Design review of the part built by this model. Coordinates are the model's own, in mm. A direction names the side the tool comes from. Coordinates: 2 decimals unless noted, no trailing zeros. Loops run counter-clockwise (first coordinate to the right, second up) from the corner with the lowest first, then second, coordinate; pieces in that order, holes last. Notation, with made-up numbers: M -31,-9 L 16,-9 A30 ccw 16,14 Z; hole C 9.5,-25.75 d11. An arc over 180 degrees is marked long. Answer as a JSON object with one key per item and string values. Group by question number.
1. Consider section B-B (z = -2.5). State the section outline as (x, y) points, then the cut area to 3 significant figures.
2. Consider section A-A (x = -17.5). State the section outline as (y, z) points.
3. To check wall thickness, follow probe 1 along X at (y, z) = (-2, -1); probe 2 along Y at (x, z) = (-17.5, -2.3); probe 3 along Z at (x, y) = (13.5, -1.25). State the ranges of each line that lie inside material, in increasing order.
4. Draft analysis for pull direction X (two halves, no side actions). For faces 1 (the flat face through (23, 0, -2)), 2 (the flat face through (-11, 1, -2)), 3 (the flat face through (20, 0, 0)), state which applies: +X half, -X half, draft (parallel to the pull), parting line (faces both ways), or undercut.
5. Insertion check: pin 1 (4.5 mm diameter, centred on x = -17.5, y = 0, fed in from -Z); pin 2 (6 mm diameter, centred on x = -16, y = -1, fed in from +Z); pin 3 (1.5 mm diameter, centred on y = -4.5, z = 1.5, fed in from +X); pin 4 (1.5 mm diameter, centred on x = 4, y = 1.5, fed in from -Z). Each pin has a flat end and moves straight along its axis. Give the tip position at first contact, or say it passes through.
6. Consider section C-C (y = 0). Count the separate pieces of the cut face and the enclosed holes in it, then the cut area to 3 significant figures.
7. Machinability: for faces 4 (the flat face through (5.432, 0.158, 1.755)), 5 (the flat face through (0, 0, 4)), 6 (the flat face through (-11, 4, -3)), 7 (the flat face through (0, -6.8, 3)), 8 (the flat face through (-8.25, -5, -1)), which of the approach directions +Z, -Z, +X, -X, +Y, -Y give a long, thin tool a straight path to every point of the face, cutting with its end or side? Answer none if there is none.
from build123d import *

# Parameters (mm, degrees)
SKETCH_W        = 46
SKETCH_H        = 13.6
SKETCH_R        = 1.7
PAD_DEPTH       = 4
PAD001_DEPTH    = 4
SKETCH002_W     = 4.3
SKETCH002_H     = 1.7
POCKET_DEPTH    = 10
SKETCH003_W     = 16.5
SKETCH003_H     = 7.2
POCKET001_DEPTH = 4
SKETCH004_W     = 3
SKETCH004_H     = 1.5
POCKET002_DEPTH = 110.862709
SKETCH005_W     = 18.5
SKETCH005_H     = 3.5
SKETCH005_W_2   = 2.5
SKETCH005_H_2   = 6
POCKET003_DEPTH = 2
CHAMFER_SIZE    = 1.99
CHAMFER001_SIZE = 1.99


with BuildPart() as part:
    # Sketch → Pad (new body)
    with BuildSketch(Plane.XY):
        Rectangle(SKETCH_W, SKETCH_H)
        with Locations((-17.5, 0)):
            Circle(SKETCH_R, mode=Mode.SUBTRACT)
        with Locations((17.5, 0)):
            Circle(SKETCH_R, mode=Mode.SUBTRACT)
    extrude(amount=-PAD_DEPTH)

    # Sketch001 → Pad001 (new body)
    with BuildSketch(Plane.XY):
        with BuildLine():
            ThreePointArc((-4.75, 6.8), (-11.55, 0), (-4.75, -6.8))
            Line((-4.75, -6.8), (4.75, -6.8))
            ThreePointArc((4.75, -6.8), (11.55, 0), (4.75, 6.8))
            Line((-4.75, 6.8), (4.75, 6.8))
        make_face()
    extrude(amount=PAD001_DEPTH)

    # Sketch002 → Pocket (cut)
    with BuildSketch(Plane.XZ.offset(6.8)):
        Polygon((-7.588114, 2.079739), (-3.336138, 1.438879), (-3.589501, -0.242134), (-7.841477, 0.398725), align=None)
        with Locations((0, 0.5)):
            Rectangle(SKETCH002_W, SKETCH002_H)
        Polygon((3.336139, 1.438884), (7.588117, 2.079734), (7.841476, 0.39872), (3.589499, -0.24213), align=None)
    extrude(amount=-POCKET_DEPTH, mode=Mode.SUBTRACT)

    # Sketch003 → Pocket001 (cut)
    with BuildSketch(Plane.XZ.offset(6.8)):
        with Locations((0, -1.1)):
            Rectangle(SKETCH003_W, SKETCH003_H)
    extrude(amount=-POCKET001_DEPTH, mode=Mode.SUBTRACT)

    # Sketch004 → Pocket002 (cut, through all)
    with BuildSketch(Plane.XZ.offset(6.8)):
        with Locations((-13, -0.75)):
            Rectangle(SKETCH004_W, SKETCH004_H)
    pocket002 = extrude(amount=-POCKET002_DEPTH, mode=Mode.SUBTRACT)

    # Mirrored: Pocket002 across Sketch004 V_Axis
    add(pocket002.mirror(Plane(origin=(0, -6.8, 0), x_dir=(0, -1, 0), z_dir=(1, 0, 0))), mode=Mode.SUBTRACT)

    # Sketch005 → Pocket003 (cut)
    with BuildSketch(Plane(origin=(0, 0, -4), x_dir=(1, 0, 0), z_dir=(0, 0, -1))):
        with Locations((0, -2.25)):
            Rectangle(SKETCH005_W, SKETCH005_H)
        with Locations((-11.3, -1)):
            Rectangle(SKETCH005_W_2, SKETCH005_H_2)
    extrude(amount=-POCKET003_DEPTH, mode=Mode.SUBTRACT)

    # Chamfer
    chamfer_edges = [part.edges().sort_by_distance(p)[0] for p in [
        (-11.3, -2, -4),
    ]]
    chamfer(chamfer_edges, length=CHAMFER_SIZE)

    # Chamfer001
    chamfer001_edges = [part.edges().sort_by_distance(p)[0] for p in [
        (0, 0.5, -4),
    ]]
    chamfer(chamfer001_edges, length=CHAMFER001_SIZE)


solid = part.part
Findings below:
{
 "1": {"outline": "M -23,-6.8 L -8.25,-6.8 L -8.25,-2.8 L 8.25,-2.8 L 8.25,-6.8 L 23,-6.8 L 23,6.8 L -23,6.8 Z; hole C -17.5,0 d3.4; hole M -12.55,-2.49 L -10.05,-2.49 L -10.05,4 L -12.55,4 Z; hole M -9.25,0.01 L 9.25,0.01 L 9.25,4 L -9.25,4 Z; hole C 17.5,0 d3.4", "area": "451 mm^2"},
 "2": {"outline": "M -6.8,-4 L -1.7,-4 L -1.7,0 L -6.8,0 Z; M 1.7,-4 L 6.8,-4 L 6.8,0 L 1.7,0 Z"},
 "3": {"probe 1": "x = -23 to -14.5, -11.5 to 11.5, 14.5 to 23", "probe 2": "y = -6.8 to -1.7, 1.7 to 6.8", "probe 3": "z = -4 to -1.5"},
 "4": {"face 1": "+X half", "face 2": "undercut", "face 3": "draft"},
 "5": {"pin 1": "stops at z = -4", "pin 2": "stops at z = 0", "pin 3": "stops at x = 10.42", "pin 4": "stops at z = -2"},
 "6": {"separate pieces": "3", "enclosed holes": "3", "area": "186 mm^2"},
 "7": {"face 4": "-Y", "face 5": "+Z, +X, -X, +Y, -Y", "face 6": "-Z", "face 7": "+Z, -Z, +X, -X, -Y", "face 8": "-Z, -Y"}
}
